Build history of the part. All positions in model axes, mm. Face numbers are marked on the shaded views. A direction names the side the tool comes from. Give positions to 0.01 mm unless a question says otherwise; leave off trailing zeros. Order: outer loops, then holes, each group sorted by start corner. A loop starts at its lowest first (then second) coordinate and runs counter-clockwise, first axis right, second up. Notation, with made-up numbers: M 30,20 L 64,20 A19 ccw 64,38 Z; hole C 44,72.5 d1. An arc over 180 degrees is marked long. Answer as CSV lines item,"result".
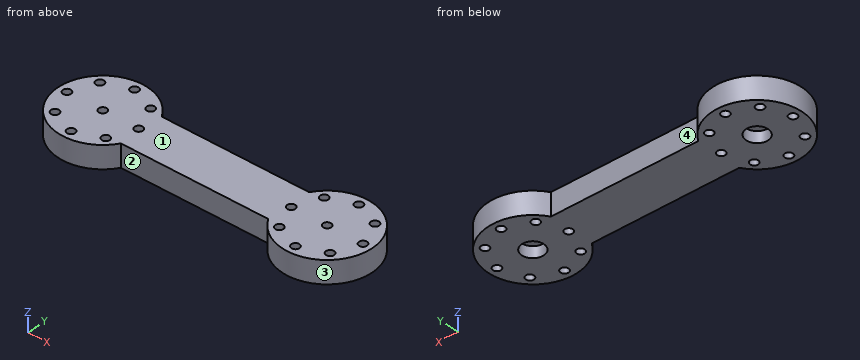
from build123d import *

# Parameters (mm, degrees)
ESQUISSE1_R             = 2.45
BOSS_EXTRU_1_DEPTH      = 5
BOSS_EXTRU_2_START      = -2.53
ESQUISSE2_R             = 2.45
ESQUISSE2_R_2           = 0.9
BOSS_EXTRU_2_DEPTH      = 2.53
BOSS_EXTRU_4_START      = -5
ESQUISSE4_R             = 10
ESQUISSE4_R_2           = 2.45
BOSS_EXTRU_4_DEPTH      = 5
ESQUISSE5_R             = 0.9
ENL_V_MAT_EXTRU_3_DEPTH = 10


with BuildPart() as part:
    # Esquisse1 → Boss.-Extru.1 (new body)
    with BuildSketch(Plane.XY):
        with BuildLine():
            Line((0, 5.147731849), (50, 5.147731849))
            ThreePointArc((50, 5.147731849), (55.147731849, 0), (50, -5.147731849))
            Line((50, -5.147731849), (0, -5.147731849))
            ThreePointArc((0, -5.147731849), (-5.147731849, 0), (0, 5.147731849))
        make_face()
        Circle(ESQUISSE1_R, mode=Mode.SUBTRACT)
        with Locations((50, 0)):
            Circle(ESQUISSE1_R, mode=Mode.SUBTRACT)
    extrude(amount=BOSS_EXTRU_1_DEPTH)

    # Esquisse2 → Boss.-Extru.2 (add)
    # profile 1 of 2: a face of its own
    with BuildSketch(Plane.XY.offset(5).offset(BOSS_EXTRU_2_START)):
        Circle(ESQUISSE2_R)
        Circle(ESQUISSE2_R_2, mode=Mode.SUBTRACT)
    # profile 2 of 2: a face of its own
    with BuildSketch(Plane.XY.offset(5).offset(BOSS_EXTRU_2_START)):
        with Locations(Location((50, 0, 0), (0, 0, 180))):
            Circle(ESQUISSE2_R)
        with Locations(Location((50, 0, 0), (0, 0, 180))):
            Circle(ESQUISSE2_R_2, mode=Mode.SUBTRACT)
    extrude(amount=BOSS_EXTRU_2_DEPTH)

    # Esquisse4 → Boss.-Extru.4 (add)
    # profile 1 of 2: a face of its own
    with BuildSketch(Plane.XY.offset(5).offset(BOSS_EXTRU_4_START)):
        Circle(ESQUISSE4_R)
        Circle(ESQUISSE4_R_2, mode=Mode.SUBTRACT)
    # profile 2 of 2: a face of its own
    with BuildSketch(Plane.XY.offset(5).offset(BOSS_EXTRU_4_START)):
        with Locations((50, 0)):
            Circle(ESQUISSE4_R)
        with Locations(Location((50, 0, 0), (0, 0, 180))):
            Circle(ESQUISSE4_R_2, mode=Mode.SUBTRACT)
    extrude(amount=BOSS_EXTRU_4_DEPTH)

    # Esquisse5 → Enlèv. mat.-Extru.3 (cut)
    with BuildSketch(Plane.XY.offset(5)):
        with Locations((-8, 0)):
            Circle(ESQUISSE5_R)
        with Locations((-5.656854249, 5.656854249)):
            Circle(ESQUISSE5_R)
        with Locations((0, 8)):
            Circle(ESQUISSE5_R)
        with Locations((5.656854249, 5.656854249)):
            Circle(ESQUISSE5_R)
        with Locations((8, 0)):
            Circle(ESQUISSE5_R)
        with Locations((5.656854249, -5.656854249)):
            Circle(ESQUISSE5_R)
        with Locations((0, -8)):
            Circle(ESQUISSE5_R)
        with Locations((-5.656854249, -5.656854249)):
            Circle(ESQUISSE5_R)
        with Locations((44.343145751, 5.656854249)):
            Circle(ESQUISSE5_R)
        with Locations((42, 0)):
            Circle(ESQUISSE5_R)
        with Locations((44.343145751, -5.656854249)):
            Circle(ESQUISSE5_R)
        with Locations((50, -8)):
            Circle(ESQUISSE5_R)
        with Locations((55.656854249, -5.656854249)):
            Circle(ESQUISSE5_R)
        with Locations((58, 0)):
            Circle(ESQUISSE5_R)
        with Locations((55.656854249, 5.656854249)):
            Circle(ESQUISSE5_R)
        with Locations((50, 8)):
            Circle(ESQUISSE5_R)
    extrude(amount=-ENL_V_MAT_EXTRU_3_DEPTH, mode=Mode.SUBTRACT)


solid = part.part
Item 1: Pull direction X, two halves, no side cores. Call the marked faces 1 and 2: released by +X, released by -X, zero draft, split by the parting line, or undercut.
Geometry says:
face 1,"zero draft"
face 2,"undercut"
Item 2: 3-axis set-ups, long thin cutter, end or side, ignore diameter. For the marked faces 3 and 4: which of +Z, -Z, +X, -X, +Y, -Y reach the whole face in a straight line?
Geometry says:
face 3,"+Z, -Z"
face 4,"+Z, -Z, +Y"
Item 3: Band-saw the part on A-A (y = -8). Give the cut face in (x, z).
Geometry says:
outline,"M -6,0 L -0.9,0 L -0.9,5 L -6,5 Z; M 0.9,0 L 6,0 L 6,5 L 0.9,5 Z; M 44,0 L 49.1,0 L 49.1,5 L 44,5 Z; M 50.9,0 L 56,0 L 56,5 L 50.9,5 Z"
Item 4: Probe line 1 along Y through (x, z) = (50, 2.6); line 2 along Y through (x, z) = (55, 0.2); line 3 along X through (y, z) = (1.25, 2.3). List the from-to ranges inside material, lowest first. Write a range as from..to.
Geometry says:
line 1,"y = -10..-8.9, -7.1..-0.9, 0.9..7.1, 8.9..10"
line 2,"y = -8.66..-6.27, -5.04..5.04, 6.27..8.66"
line 3,"x = -9.92..-2.11, 2.11..47.89, 52.11..59.92"
Item 5: Drop flat-ended pins along their axis: pin 1 (1.6 mm diameter, centred on x = 42, y = 0, fed in from -Z); pin 2 (2 mm diameter, centred on x = 0, y = 0, fed in from -Z); pin 3 (2.5 mm diameter, centred on x = 27, z = 3.5, fed in from -Y); pin 4 (1.5 mm diameter, centred on y = 7.5, z = 2, fed in from +X). Give the stop position or say it passes through.
Geometry says:
pin 1,"passes through"
pin 2,"stops at z = 2.47"
pin 3,"stops at y = -5.15"
pin 4,"stops at x = 57.38"
Item 6: Band-saw the part on D-D (z = 0.95). State how many separate pieces and enclosed holes the cut face has, and give its area (3 significant figures).
Geometry says:
separate pieces,"1"
enclosed holes,"18"
area,"868 mm2"
Item 7: Band-saw the part on B-B (x = 58). Give the cut face in (y, z), and give its area (3 significant figures).
Geometry says:
outline,"M -6,0 L -0.9,0 L -0.9,5 L -6,5 Z; M 0.9,0 L 6,0 L 6,5 L 0.9,5 Z"
area,"51.0 mm2"
Item 8: Band-saw the part on C-C (x = 0). Give the cut face in (y, z), and give its area (3 significant figures).
Geometry says:
outline,"M -10,0 L -8.9,0 L -8.9,5 L -10,5 Z; M -7.1,0 L -2.45,0 L -2.45,2.47 L -0.9,2.47 L -0.9,5 L -7.1,5 Z; M 0.9,2.47 L 2.45,2.47 L 2.45,0 L 7.1,0 L 7.1,5 L 0.9,5 Z; M 8.9,0 L 10,0 L 10,5 L 8.9,5 Z"
area,"65.3 mm2"
